Could you check a few things on this model? Use its own coordinates, in mm. A direction names the side the tool comes from. Round coordinates to 2 decimals unless told otherwise and drop trailing zeros. Loops run counter-clockwise (first coordinate to the right, second up) from the corner with the lowest first, then second, coordinate; pieces in that order, holes last. Notation, with made-up numbers: (36.25, 32.5) -> (49.25, 32.5) arc R18 cw to (49.25, 37.5) -> close; hole circle Ø10 at (8.5, 8). An arc over 180 degrees is marked (long way). Use CSV: the item, a comma, the result in double quotes. Start each with the question number.
```python
from build123d import *

# Parameters (mm, degrees)
SKETCH1_W           = 6
SKETCH1_H           = 6
BOSS_EXTRUDE1_DEPTH = 9
CUT_EXTRUDE1_DEPTH  = 3
SKETCH3_W           = 1
SKETCH3_H           = 2
CUT_EXTRUDE2_DEPTH  = 1
CUT_EXTRUDE3_DEPTH  = 1
SKETCH5_W           = 2
SKETCH5_H           = 1
CUT_EXTRUDE4_DEPTH  = 3
SKETCH6_W           = 1
SKETCH6_H           = 3
CUT_EXTRUDE5_DEPTH  = 2
CUT_EXTRUDE6_DEPTH  = 2


with BuildPart() as part:
    # Sketch1 → Boss-Extrude1 (new body)
    with BuildSketch(Plane.XY):
        Rectangle(SKETCH1_W, SKETCH1_H)
    extrude(amount=BOSS_EXTRUDE1_DEPTH)

    # Sketch2 → Cut-Extrude1 (cut)
    with BuildSketch(Plane(origin=(0, 3, 0), x_dir=(1, 0, 0), z_dir=(0, 1, 0))):
        Polygon((1, 0), (-1, 0), (-1, -2), (-2, -2), (-2, -7), (1, -7), (1, -9), (3, -9), (3, -6), (1, -6), align=None)
    extrude(amount=-CUT_EXTRUDE1_DEPTH, mode=Mode.SUBTRACT)

    # Sketch3 → Cut-Extrude2 (cut)
    with BuildSketch(Plane(origin=(0, 3, 0), x_dir=(1, 0, 0), z_dir=(0, 1, 0))):
        with Locations((-2.5, -4)):
            Rectangle(SKETCH3_W, SKETCH3_H)
    extrude(amount=-CUT_EXTRUDE2_DEPTH, mode=Mode.SUBTRACT)

    # Sketch4 → Cut-Extrude3 (cut)
    with BuildSketch(Plane.ZY.offset(3)):
        Polygon((7, 3), (9, 0), (9, 3), align=None)
    extrude(amount=-CUT_EXTRUDE3_DEPTH, mode=Mode.SUBTRACT)

    # Sketch5 → Cut-Extrude4 (cut)
    with BuildSketch(Plane(origin=(1, 0, 0), x_dir=(0, 0, -1), z_dir=(1, 0, 0))):
        with Locations((-8, 2.5)):
            Rectangle(SKETCH5_W, SKETCH5_H)
    extrude(amount=-CUT_EXTRUDE4_DEPTH, mode=Mode.SUBTRACT)

    # Sketch6 → Cut-Extrude5 (cut)
    with BuildSketch(Plane(origin=(3, 0, 0), x_dir=(0, 0, -1), z_dir=(1, 0, 0))):
        with Locations((-8.5, -1.5)):
            Rectangle(SKETCH6_W, SKETCH6_H)
    extrude(amount=-CUT_EXTRUDE5_DEPTH, mode=Mode.SUBTRACT)

    # Sketch7 → Cut-Extrude6 (cut)
    with BuildSketch(Plane(origin=(3, 0, 0), x_dir=(0, 0, -1), z_dir=(1, 0, 0))):
        Polygon((-1, 3), (-6, 1), (-6, 3), align=None)
    extrude(amount=-CUT_EXTRUDE6_DEPTH, mode=Mode.SUBTRACT)


solid = part.part
```
1. We'd pull the mould along X, two halves only. Please class faces 1 (the face through (-2.5, 3, 6)), 2 (the face through (-1, 2, 1)), 3 (the face through (3, -1, 3)): pulls with the +X half, pulls with the -X half, needs draft (parallel to the pull), parting line crosses it, or undercut.
2. Will these pins go through, and if not, where does the flat tip stop? pin 1 (1.1 mm diameter, centred on x = 2, y = 0.5, fed in from +Z); pin 2 (1.6 mm diameter, centred on x = 0, y = 1.5, fed in from -Z); pin 3 (1.6 mm diameter, centred on x = -1, z = 8.5, fed in from +Y).
3. Suppose I cut it at B-B (z = 4.75). List the corners of the cut face in (x, y) for me, then the cut area to 3 significant figures.
4. Suppose I cut it at C-C (x = -1.9). List the corners of the cut face in (y, z) for me.
5. If I drill on L1, parallel to Z at x = -1.3, y = 0.8; L2, parallel to Y at x = -0.4, z = 3.75; L3, parallel to Z at x = -1.1, y = 2.1, over which ranges is the centre line in solid material (lowest first)?
6. Suppose I cut it at A-A (y = 1.2). List the corners of the cut face in (x, z) for me.
7. For faces 4 (the face through (-2.5, 2, 4)), 5 (the face through (-1.5, 1.5, 2)), 6 (the face through (2, 2, 3.5)), which set-ups out of +Z, -Z, +X, -X, +Y, -Y let a thin tool reach every point of the face, with its end or its side?
8. Suppose I cut it at D-D (y = 2.3). List the corners of the cut face in (x, z) for me.
Geometry check:
1,face 1,"needs draft"
1,face 2,"undercut"
1,face 3,"pulls with the +X half"
2,pin 1,"stops at z = 8"
2,pin 2,"stops at z = 7"
2,pin 3,"stops at y = 2"
3,outline,"(-3, -3) -> (3, -3) -> (3, 1.5) -> (1, 1.5) -> (1, 0) -> (-2, 0) -> (-2, 2) -> (-3, 2) -> close"
3,area,"23.0 mm²"
4,outline,"(-3, 0) -> (3, 0) -> (3, 2) -> (0, 2) -> (0, 7) -> (2, 7) -> (2, 9) -> (-3, 9) -> close"
5,L1,"z = 0 to 2, 7 to 9"
5,L2,"y = -3 to 0"
5,L3,"z = 0 to 2"
6,outline,"(-3, 0) -> (-1, 0) -> (-1, 2) -> (-2, 2) -> (-2, 7) -> (1, 7) -> (1, 9) -> (-2, 9) -> (-2, 8.2) -> (-3, 8.2) -> close; (1, 0) -> (3, 0) -> (3, 5.5) -> (1, 5.5) -> close"
7,face 4,"-X, +Y"
7,face 5,"+Y"
7,face 6,"+Z, +X, +Y"
8,outline,"(-3, 0) -> (-1, 0) -> (-1, 2) -> (-2, 2) -> (-2, 3) -> (-3, 3) -> close; (-3, 5) -> (-2, 5) -> (-2, 7.47) -> (-3, 7.47) -> close; (1, 0) -> (3, 0) -> (3, 2.75) -> (1, 2.75) -> close"
